For this review, take the finished solid that the model builds, in its own axes (mm). A direction names the side the tool comes from. Round coordinates to 2 decimals unless told otherwise and drop trailing zeros. Write each loop counter-clockwise with the first axis right and the second up, starting at its lowest first coordinate (ties: lowest second). Pieces come first, ordered by that corner, then holes. Notation, with made-up numbers: (70.5, -31.75) -> (125.5, -31.75) arc R16 cw to (125.5, -20.75) -> close; hole circle Ø5 at (83.5, 3). An arc over 180 degrees is marked (long way). Answer as CSV lines item,"result". Start each with the question number.
Item 1: Mouldability with a two-part tool opening along X and no side actions: class faces 1 (the flat face through (-63.34, 18.01, 1.52)), 2 (the flat face through (59.42, -18.99, 1.52)), 3 (the cylindrical face through (94.91, -14.21, 1.48)), 4 (the cylindrical face through (-94.969, 14.136, 1.479)) as +X half, -X half, draft (parallel to the pull), parting line (faces both ways), or undercut.
Item 2: Take a section at B-B on z = 1.75. Count the separate pieces of the cut face and the enclosed holes in it, then the cut area to 3 significant figures.
Item 3: Machinability: for faces 5 (the flat face through (-44.363, 12.371, 1.521)), 6 (the flat face through (-1, 0, 0)), which of the approach directions +Z, -Z, +X, -X, +Y, -Y give a long, thin tool a straight path to every point of the face, cutting with its end or side? Answer none if there is none.
Item 4: Wall thickness on probe 1 along Y at (x, z) = (-31, 1); probe 2 along Y at (x, z) = (-60, 1.1); probe 3 along Y at (x, z) = (16, 1.05): over which ranges is each line inside the solid? List them lowest first. Write a range as from..to.
Item 5: Take a section at A-A on x = 49.5. Give the boundary of the cut face in (y, z) (3 decimals), then the cut area to 3 significant figures.
```python
from build123d import *

# Parameters (mm, degrees)
SKETCH_1_W          = 202
SKETCH_1_H          = 60
SKETCH_1_R          = 1.35
EXTRUDE_1_DEPTH     = 3
SKETCH_2_R          = 1.6
CUT_EXTRUDE_1_DEPTH = 10
SKETCH_3_OUTSIDE_W  = 246.148
SKETCH_3_OUTSIDE_H  = 104.148
CUT_EXTRUDE_2_DEPTH = 10
CUT_EXTRUDE_3_DEPTH = 10
CUT_EXTRUDE_4_DEPTH = 10
FILLET_1_R          = 2
FILLET_2_R          = 5


with BuildPart() as part:
    # 草图1 → 凸台-拉伸1 (new body)
    with BuildSketch(Plane.XY):
        Rectangle(SKETCH_1_W, SKETCH_1_H)
        with Locations((31, 25)):
            Circle(SKETCH_1_R, mode=Mode.SUBTRACT)
        with Locations((-31, 25)):
            Circle(SKETCH_1_R, mode=Mode.SUBTRACT)
        with Locations((-31, -25)):
            Circle(SKETCH_1_R, mode=Mode.SUBTRACT)
        with Locations((31, -25)):
            Circle(SKETCH_1_R, mode=Mode.SUBTRACT)
    extrude(amount=EXTRUDE_1_DEPTH)

    # 草图2 → 切除-拉伸1 (cut)
    with BuildSketch(Plane.XY.offset(3)):
        with Locations((91, -10)):
            Circle(SKETCH_2_R)
        with Locations((91, 10)):
            Circle(SKETCH_2_R)
    cut_extrude_1 = extrude(amount=-CUT_EXTRUDE_1_DEPTH, mode=Mode.SUBTRACT)

    # 镜向1: 切除-拉伸1 across plane
    add(cut_extrude_1.mirror(Plane(origin=(0, 0, 0), x_dir=(0, 0, 1), z_dir=(1, 0, 0))), mode=Mode.SUBTRACT)

    # 草图3 outside → 切除-拉伸2 (cut)
    with BuildSketch(Plane.XY.offset(3)):
        Rectangle(SKETCH_3_OUTSIDE_W, SKETCH_3_OUTSIDE_H)
        Polygon((-96, 15), (-96, -15), (-36, -30), (36, -30), (96, -15), (96, 15), (36, 30), (-36, 30), align=None, mode=Mode.SUBTRACT)
    extrude(amount=-CUT_EXTRUDE_2_DEPTH, mode=Mode.SUBTRACT)

    # 草图4 → 切除-拉伸3 (cut)
    with BuildSketch(Plane.XY.offset(3)):
        Polygon((-32.5, 25.721117968), (-86, 12.346117968), (-86, -12.346117968), (-57.616230147, 7.849987896), align=None)
        Polygon((-58.330965527, 2.432194903), (-80.89439135, -13.622520131), (-35.767539705, -24.904233042), align=None)
        Polygon((-32.5, -22.579257249), (-32.5, 20.811885729), (-55.063425822, 4.757170695), align=None)
    cut_extrude_3 = extrude(amount=-CUT_EXTRUDE_3_DEPTH, mode=Mode.SUBTRACT)

    # 镜向2: 切除-拉伸3 across plane
    add(cut_extrude_3.mirror(Plane(origin=(0, 0, 0), x_dir=(0, 0, 1), z_dir=(1, 0, 0))), mode=Mode.SUBTRACT)

    # 草图6 → 切除-拉伸4 (cut)
    with BuildSketch(Plane.XY.offset(3)):
        Polygon((-26, 21.531790616), (-26, -21.531790616), (-3.606937759, 0), align=None)
        Polygon((-22.393062241, 25), (0, 3.468209384), (22.393062241, 25), align=None)
        Polygon((26, 21.531790616), (3.606937759, 0), (26, -21.531790616), align=None)
        Polygon((0, -3.468209384), (-22.393062241, -25), (22.393062241, -25), align=None)
    extrude(amount=-CUT_EXTRUDE_4_DEPTH, mode=Mode.SUBTRACT)

    # 圆角1
    fillet_1_edges = [part.edges().sort_by_distance(p)[0] for p in [
        (-55.063425822, 4.757170695, 1.5),
        (-32.5, 20.811885729, 1.5),
        (-32.5, -22.579257249, 1.5),
        (-58.330965527, 2.432194903, 1.5),
        (-35.767539705, -24.904233042, 1.5),
        (-80.89439135, -13.622520131, 1.5),
        (-32.5, 25.721117968, 1.5),
        (-86, -12.346117968, 1.5),
        (-86, 12.346117968, 1.5),
        (32.5, 20.811885729, 1.5),
        (55.063425822, 4.757170695, 1.5),
        (32.5, -22.579257249, 1.5),
        (35.767539705, -24.904233042, 1.5),
        (58.330965527, 2.432194903, 1.5),
        (80.89439135, -13.622520131, 1.5),
        (86, -12.346117968, 1.5),
        (32.5, 25.721117968, 1.5),
        (86, 12.346117968, 1.5),
        (3.606937759, 0, 1.5),
        (26, 21.531790616, 1.5),
        (26, -21.531790616, 1.5),
        (0, 3.468209384, 1.5),
        (-22.393062241, 25, 1.5),
        (22.393062241, 25, 1.5),
        (-22.393062241, -25, 1.5),
        (0, -3.468209384, 1.5),
        (22.393062241, -25, 1.5),
        (-26, -21.531790616, 1.5),
        (-26, 21.531790616, 1.5),
        (-3.606937759, 0, 1.5),
    ]]
    fillet(fillet_1_edges, radius=FILLET_1_R)

    # 圆角2
    fillet_2_edges = [part.edges().sort_by_distance(p)[0] for p in [
        (-36, -30, 1.5),
        (36, -30, 1.5),
        (36, 30, 1.5),
        (-36, 30, 1.5),
        (96, 15, 1.5),
        (96, -15, 1.5),
        (-96, -15, 1.5),
        (-96, 15, 1.5),
    ]]
    fillet(fillet_2_edges, radius=FILLET_2_R)


solid = part.part
```
Output values:
1,face 1,"undercut"
1,face 2,"undercut"
1,face 3,"+X half"
1,face 4,"-X half"
2,separate pieces,"1"
2,enclosed holes,"18"
2,area,"4,570 mm^2"
3,face 5,"+Z, -Z"
3,face 6,"-Z, +X, -X, +Y, -Y"
4,probe 1,"y = -30..-26.35, -23.65..23.65, 26.35..30"
4,probe 2,"y = -24..-18.85, 1.24..6.15, 18.85..24"
4,probe 3,"y = -30..-25, -18.85..-11.92, 11.92..18.85, 25..30"
5,outline,"(-26.625, 0) -> (-21.471, 0) -> (-21.471, 3) -> (-26.625, 3) -> close; (-8.267, 0) -> (-1.983, 0) -> (-1.983, 3) -> (-8.267, 3) -> close; (8.716, 0) -> (13.625, 0) -> (13.625, 3) -> (8.716, 3) -> close; (21.471, 0) -> (26.625, 0) -> (26.625, 3) -> (21.471, 3) -> close"
5,area,"64.5 mm^2"
